from build123d import *

# Parameters (mm, degrees)
SKETCH_1_W          = 240
SKETCH_1_H          = 60
EXTRUDE_1_DEPTH     = 10
SKETCH_2_W          = 129.92
SKETCH_2_H          = 10
CUT_EXTRUDE_2_DEPTH = 10
SKETCH_3_R          = 4
CUT_EXTRUDE_3_DEPTH = 10


with BuildPart() as part:
    # 草图1 → 凸台-拉伸1 (new body)
    with BuildSketch(Plane.XY):
        Rectangle(SKETCH_1_W, SKETCH_1_H)
    extrude(amount=EXTRUDE_1_DEPTH)

    # 草图2 → 切除-拉伸2 (cut)
    with BuildSketch(Plane.XY.offset(10)):
        Polygon((90, 30), (19.92, 30), (90, 21.9089023), align=None)
        with BuildLine():
            Line((90, 30), (90, 21.9089023))
            ThreePointArc((90, 21.9089023), (110.564659966, 18.574175621), (120, 0))
            Line((120, 0), (120, 30))
            Line((120, 30), (90, 30))
        make_face()
        with BuildLine():
            ThreePointArc((120, 0), (110.564659966, -18.574175621), (90, -21.9089023))
            Line((90, -21.9089023), (90, -30))
            Line((90, -30), (120, -30))
            Line((120, -30), (120, 0))
        make_face()
        Polygon((90, -21.9089023), (19.92, -30), (90, -30), align=None)
        with Locations((-55.04, 25)):
            Rectangle(SKETCH_2_W, SKETCH_2_H)
        with Locations((-55.04, -25)):
            Rectangle(SKETCH_2_W, SKETCH_2_H)
    extrude(amount=-CUT_EXTRUDE_2_DEPTH, mode=Mode.SUBTRACT)

    # 草图3 → 切除-拉伸3 (cut)
    with BuildSketch(Plane.XY.offset(10)):
        with Locations((96, 0)):
            Circle(SKETCH_3_R)
    extrude(amount=-CUT_EXTRUDE_3_DEPTH, mode=Mode.SUBTRACT)


solid = part.part
Read the model definition and answer for the solid it produces. Units are mm, in the model's axes. A direction names the side the tool comes from. Round coordinates to 2 decimals unless told otherwise and drop trailing zeros. Write each loop counter-clockwise with the first axis right and the second up, starting at its lowest first coordinate (ties: lowest second). Pieces come first, ordered by that corner, then holes. Notation, with made-up numbers: M -15.75,-34 L -0.75,-34 A26 cw -0.75,-13 Z; hole C 25.25,53 d6. An arc over 180 degrees is marked long. Use a Markdown table: item, result.
1) The part is cut by section A-A (z = 7.75). Write down the section's boundary in (x, y).
Answers follow:
| item | result |
|---|---|
| outline | M -120,-20 L 9.92,-20 L 9.92,-30 L 19.92,-30 L 90,-21.91 A23 ccw long 90,21.91 L 19.92,30 L 9.92,30 L 9.92,20 L -120,20 Z; hole C 96,0 d8 |
2) For a pull along X with two mould halves and no side action, classify faces 4 (the cylindrical face through (92, 0, 5)), 5 (the flat face through (-2, 0, 10)), 6 (the flat face through (-120, 0, 5)) as pulls with the +X half, pulls with the -X half, needs draft (parallel to the pull), parting line crosses it, or undercut.
Answers follow:
| item | result |
|---|---|
| face 4 | undercut |
| face 5 | needs draft |
| face 6 | pulls with the -X half |
3) Straight lines are drawn through the part: line 1 along Y through (x, z) = (96, 8); line 2 along Y through (x, z) = (-89, 5); line 3 along Y through (x, z) = (85.5, 8.25). For each, find the intervals that lie inside material, in ascending order. Write a range as [from, to].
Answers follow:
| item | result |
|---|---|
| line 1 | y = [-22.98, -4], [4, 22.98] |
| line 2 | y = [-20, 20] |
| line 3 | y = [-22.43, 22.43] |
4) The part is cut by section C-C (x = -70). Write down the section's boundary in (y, z), plus the area to 3 significant figures.
Answers follow:
| item | result |
|---|---|
| outline | M -20,0 L 20,0 L 20,10 L -20,10 Z |
| area | 400 mm2 |
5) Flat-ended cylindrical pins translate along their axes: pin 1 (5 mm diameter, centred on x = 42, z = 4.5, fed in from +Y); pin 2 (5 mm diameter, centred on x = -43.5, z = 6, fed in from -Y); pin 3 (1 mm diameter, centred on y = 16, z = 7, fed in from +X). Find the tip coordinate at first contact, or state that the pin passes through.
Answers follow:
| item | result |
|---|---|
| pin 1 | stops at y = 27.74 |
| pin 2 | stops at y = -20 |
| pin 3 | stops at x = 113.99 |
6) The part is cut by section D-D (y = 13). Write down the section's boundary in (x, z).
Answers follow:
| item | result |
|---|---|
| outline | M -120,0 L 115.97,0 L 115.97,10 L -120,10 Z |
7) A tool of negligible diameter and unlimited length cuts with its end or side. For faces 1 (the flat face through (-56, 20, 5)), 2 (the flat face through (15, -30, 5)), 3 (the flat face through (9.92, -25, 5)), from which of +Z, -Z, +X, -X, +Y, -Y can it reach the whole face along a straight path? Write none if from no direction.
Answers follow:
| item | result |
|---|---|
| face 1 | +Z, -Z, -X, +Y |
| face 2 | +Z, -Z, +X, -X, -Y |
| face 3 | +Z, -Z, -X, -Y |
8) The part is cut by section B-B (x = 96). Write down the section's boundary in (y, z), plus the area to 3 significant figures.
Answers follow:
| item | result |
|---|---|
| outline | M -22.98,0 L -4,0 L -4,10 L -22.98,10 Z; M 4,0 L 22.98,0 L 22.98,10 L 4,10 Z |
| area | 380 mm2 |
